Could you check a few things on this model? Use its own coordinates, in mm. Give positions to 0.01 mm unless a question says otherwise; leave off trailing zeros. Loops run counter-clockwise (first coordinate to the right, second up) from the corner with the lowest first, then second, coordinate; pieces in that order, holes last.
1. Thinking about a two-plate mould opening in X: for faces 1 (the flat face through (-2, 0, 2)), 2 (the cylindrical face through (0, 3, -2)), 3 (the cylindrical face through (-7.493, 3.357, 0.33)), which applies, +X half, -X half, draft (parallel to the pull), parting line (faces both ways), or undercut?
2. Imagine slicing it at C-C (y = 2). List the corners of the cut face in (x, z) for me.
3. Imagine slicing it at B-B (z = 0). List the corners of the cut face in (x, y) for me.
4. I need wall thicknesses on line 1 along Z through (x, y) = (0, 2); line 2 along Z through (x, y) = (0.5, 4.25); line 3 along Z through (x, y) = (-4.5, 1.75). Which ranges of each line are inside material? Lowest first, please.
5. For P1, Ø6, axis at x = -4.5, z = -1.5, coming from the -Y side; P2, Ø1, axis at y = 2.5, z = 1, coming from the -X side; P3, Ø1.5, axis at x = -5, y = 4.5, coming from the -Z side; P4, Ø2.5, axis at x = 0, z = 0, coming from the -Y side, each with a flat end and sliding along its axis, tell me the tip position at first contact or that it passes through.
6. Imagine slicing it at A-A (x = 0). List the corners of the cut face in (y, z) for me.
```python
from build123d import *

# Parameters (mm, degrees)
F0_R     = 7.5
F1_DEPTH = 6.8
F2_R     = 2
F3_DEPTH = 24.4
F4_R     = 0.3
F5_R     = 0.3


with BuildPart() as f1:
    # F0 (on Front) → F1 (new body)
    with BuildSketch(Plane.XZ):
        Circle(F0_R)
    extrude(amount=-F1_DEPTH)

    # F2 (on face) → F3 (cut)
    with BuildSketch(Plane.XZ):
        Circle(F2_R)
    extrude(amount=-F3_DEPTH, mode=Mode.SUBTRACT)

    # F4
    f4_edges = [f1.edges().sort_by_distance(p)[0] for p in [
        (-7.5, 0, 0),
        (-2, 0, 0),
        (-7.5, 6.8, 0),
    ]]
    fillet(f4_edges, radius=F4_R)

    # F5
    f5_edges = [f1.edges().sort_by_distance(p)[0] for p in [
        (-2, 6.8, 0),
    ]]
    fillet(f5_edges, radius=F5_R)


solid = f1.part
```
Derived:
1. face 1: draft
1. face 2: undercut
1. face 3: parting line
2. outline: circle Ø15 at (0, 0); hole circle Ø4 at (0, 0)
3. outline: (-7.5, 0.3) arc R0.3 ccw to (-7.2, 0) - (-2.3, 0) arc R0.3 ccw to (-2, 0.3) - (-2, 6.5) arc R0.3 ccw to (-2.3, 6.8) - (-7.2, 6.8) arc R0.3 ccw to (-7.5, 6.5) - close; (2, 0.3) arc R0.3 ccw to (2.3, 0) - (7.2, 0) arc R0.3 ccw to (7.5, 0.3) - (7.5, 6.5) arc R0.3 ccw to (7.2, 6.8) - (2.3, 6.8) arc R0.3 ccw to (2, 6.5) - close
4. line 1: z = -7.5 to -2, 2 to 7.5
4. line 2: z = -7.48 to -1.94, 1.94 to 7.48
4. line 3: z = -6 to 6
5. P1: stops at y = 0
5. P2: stops at x = -7.48
5. P3: stops at z = -6.18
5. P4: passes through
6. outline: (0, -7.2) arc R0.3 ccw to (0.3, -7.5) - (6.5, -7.5) arc R0.3 ccw to (6.8, -7.2) - (6.8, -2.3) arc R0.3 ccw to (6.5, -2) - (0.3, -2) arc R0.3 ccw to (0, -2.3) - close; (0, 2.3) arc R0.3 ccw to (0.3, 2) - (6.5, 2) arc R0.3 ccw to (6.8, 2.3) - (6.8, 7.2) arc R0.3 ccw to (6.5, 7.5) - (0.3, 7.5) arc R0.3 ccw to (0, 7.2) - close
